Could you check a few things on this model? Use its own coordinates, in mm. A direction names the side the tool comes from. Give positions to 0.01 mm unless a question says otherwise; leave off trailing zeros. Order: outer loops, then holes, each group sorted by start corner. A loop starts at its lowest first (then second) coordinate and runs counter-clockwise, first axis right, second up. Notation, with made-up numbers: M 56.25,33.25 L 110.25,33.25 A24 ccw 110.25,54.25 Z; hole C -23.75,-23 d7. An arc over 180 degrees is marked long. Use a Markdown table: item, result. Add a question column.
Item 1: If I drill on L1, parallel to Y at x = -15, z = 11.5; L2, parallel to X at y = -0.25, z = 0.5; L3, parallel to X at y = -2.25, z = 13, over which ranges is the centre line in solid material (lowest first)? Write a range as from..to.
Item 2: I'm going to push a flat-ended pin straight in: pin 1 Ø4 at (x, y) = (7, -2.5) entering from +Z. Where does the tip first touch, or does it pass through?
Item 3: Suppose I cut it at C-C on y = -8.5. Write out the boundary of the cut face in (x, z), plus the area to 3 significant figures.
Item 4: If we mould it in two halves opening along X, with no side actions, what happens to faces 3 (the face through (12.5, -2.4, 7.6)), 4 (the face through (8.83, -2.36, 14.21)), 5 (the face through (0, 0, 0)), 6 (the face through (-22, 0, 7))? For each: released by +X, released by -X, zero draft, split by the parting line, or undercut.
Item 5: Suppose I cut it at B-B on y = -2.5. Write out the boundary of the cut face in (x, z).
Item 6: Suppose I cut it at A-A on x = -17. Write out the boundary of the cut face in (y, z), plus the area to 3 significant figures.
Item 7: Suppose I cut it at D-D on z = 1. Write out the boundary of the cut face in (x, y).
Item 8: For faces 1 (the face through (0, 12.5, 7)), 2 (the face through (-8.83, -2.36, 14.21)), which set-ups out of +Z, -Z, +X, -X, +Y, -Y let a thin tool reach every point of the face, with its end or its side?
from build123d import *

# Parameters (mm, degrees)
F0_W        = 44
F0_H        = 25
F1_DEPTH    = 15
F2_R        = 8
F3_DEPTH    = 20
F4_R        = 2.5
F5_DEPTH    = 15
F6_T1_DEPTH = 24.6515369414


# Not quite as in the source:
# - a fillet or chamfer that OpenCascade refuses, or shapes differently, is made with other operations: its cross-section is extruded or revolved along the edge and cut away or added


with BuildPart() as f1:
    # F0 (on Top) → F1 (new body)
    with BuildSketch(Plane.XY):
        Rectangle(F0_W, F0_H)
    extrude(amount=F1_DEPTH)

    # F2 (on face) → F3 (cut)
    with BuildSketch(Plane.XZ.offset(12.5)):
        with Locations((0, 15)):
            Circle(F2_R)
    extrude(amount=-F3_DEPTH, mode=Mode.SUBTRACT)

    # F4 (on face) → F5 (cut)
    with BuildSketch(Plane.XY.offset(15)):
        with Locations((-15, -2.5)):
            Circle(F4_R)
        with Locations((15, -2.5)):
            Circle(F4_R)
    extrude(amount=-F5_DEPTH, mode=Mode.SUBTRACT)

    # F6: chamfer of 2 on 2 edges, made by hand

    # F6_s2 → F6_t1 (cut)
    with BuildSketch(Plane.XZ.offset(-7.5)):
        with BuildLine():
            Line((9.7979589711, 15), (7.8383671769, 13.4))
            ThreePointArc((7.8383671769, 13.4), (7.9565711479, 14.1675484588), (8, 15))
            Line((8, 15), (9.7979589711, 15))
        make_face()
        with BuildLine():
            Line((-9.7979589711, 15), (-7.8383671769, 13.4))
            ThreePointArc((-7.8383671769, 13.4), (-7.9565711479, 14.1675484588), (-8, 15))
            Line((-8, 15), (-9.7979589711, 15))
        make_face()
    extrude(amount=F6_T1_DEPTH, mode=Mode.SUBTRACT)


solid = f1.part
Findings below:
| question | item | result |
|---|---|---|
| 1 | L1 | y = -12.5..-5, 0..12.5 |
| 1 | L2 | x = -22..-16.09, -13.91..13.91, 16.09..22 |
| 1 | L3 | x = -22..-17.49, -12.51..-7.75, 7.75..12.51, 17.49..22 |
| 2 | pin 1 | stops at z = 14.35 |
| 3 | outline | M -22,0 L 22,0 L 22,15 L 9.8,15 L 7.84,13.4 A8 cw -7.84,13.4 L -9.8,15 L -22,15 Z |
| 3 | area | 557 mm^2 |
| 4 | face 3 | undercut |
| 4 | face 4 | undercut |
| 4 | face 5 | zero draft |
| 4 | face 6 | released by -X |
| 5 | outline | M -22,0 L -17.5,0 L -17.5,15 L -22,15 Z; M -12.5,0 L 12.5,0 L 12.5,15 L 9.8,15 L 7.84,13.4 A8 cw -7.84,13.4 L -9.8,15 L -12.5,15 Z; M 17.5,0 L 22,0 L 22,15 L 17.5,15 Z |
| 6 | outline | M -12.5,0 L -4,0 L -4,15 L -12.5,15 Z; M -1,0 L 12.5,0 L 12.5,15 L -1,15 Z |
| 6 | area | 330 mm^2 |
| 7 | outline | M -22,-12.5 L 22,-12.5 L 22,12.5 L -22,12.5 Z; hole C -15,-2.5 d5; hole C 15,-2.5 d5 |
| 8 | face 1 | +Z, -Z, +X, -X, +Y |
| 8 | face 2 | +Z, -Y |
